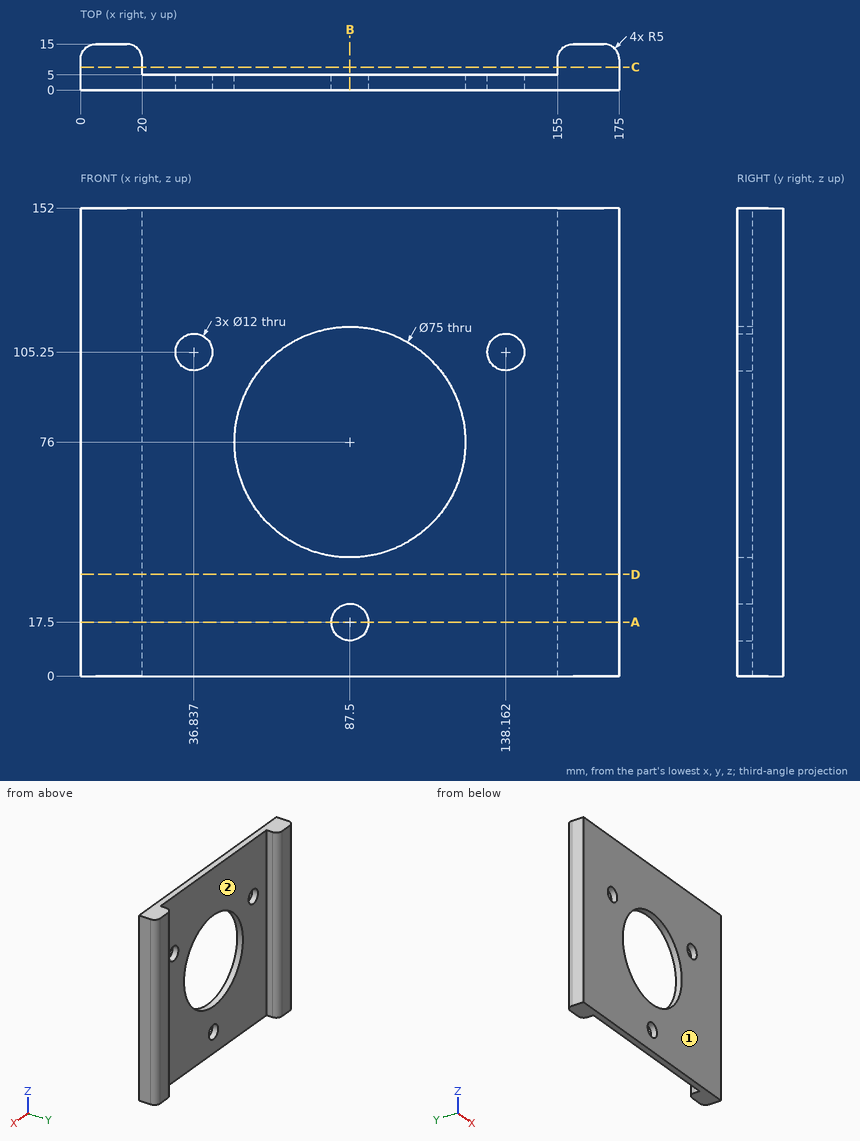
Answer from the drawing. Dimensions are ordinates in mm from the lowest x, y and z of the part. Coordinates: 2 decimals unless noted, no trailing zeros. Write each loop counter-clockwise with the first axis right and the second up, starting at its lowest first coordinate (ties: lowest second). Pieces come first, ordered by that corner, then holes. Notation, with made-up numbers: (15, 21) - (42, 21) arc R9 cw to (42, 31) - close; hole circle Ø8 at (-12.75, -28.5). An arc over 180 degrees is marked (long way). Return JSON: item names as keys, results as strings. Group by question number.
Q1. The part is cut by section D-D on z = 33. Write down the section's boundary in (x, y), and give its area (3 significant figures).
Q2. Find the intervals of material crossed by line 1 along Z through (x, y) = (87.5, 2.9); line 2 along X through (y, z) = (2.85, 105.25) (1 decimal); line 3 along X through (y, z) = (3.3, 17.5), in increasing order. Write a range as [from, to].
Q3. The part is cut by section B-B on x = 87.5. Write down the section's boundary in (y, z).
Q4. For a pull along X with two mould halves and no side action, classify the marked faces 1 and 2 as +X half, -X half, draft (parallel to the pull), parting line (faces both ways), or undercut.
Q5. The part is cut by section C-C on y = 7.5. Write down the section's boundary in (x, z).
Q6. The part is cut by section A-A on z = 17.5. Write down the section's boundary in (x, y), and give its area (3 significant figures).
Q7. Flat-ended cylindrical pins translate along their axes: pin 1 Ø15.5 at (x, z) = (138.16, 105.25) entering from +Y; pin 2 Ø9.5 at (x, z) = (36.84, 105.25) entering from -Y. Find the tip coordinate at first contact, or state that the pin passes through.
Evaluation:
{
 "1": {"outline": "(0, 0) - (175, 0) - (175, 10) arc R5 ccw to (170, 15) - (160, 15) arc R5 ccw to (155, 10) - (155, 5) - (20, 5) - (20, 10) arc R5 ccw to (15, 15) - (5, 15) arc R5 ccw to (0, 10) - close", "area": "1,250 mm2"},
 "2": {"line 1": "z = [0, 11.5], [23.5, 38.5], [113.5, 152]", "line 2": "x = [0, 30.8], [42.8, 64], [111, 132.2], [144.2, 175]", "line 3": "x = [0, 81.5], [93.5, 175]"},
 "3": {"outline": "(0, 0) - (5, 0) - (5, 11.5) - (0, 11.5) - close; (0, 23.5) - (5, 23.5) - (5, 38.5) - (0, 38.5) - close; (0, 113.5) - (5, 113.5) - (5, 152) - (0, 152) - close"},
 "4": {"face 1": "draft", "face 2": "undercut"},
 "5": {"outline": "(0, 0) - (20, 0) - (20, 152) - (0, 152) - close; (155, 0) - (175, 0) - (175, 152) - (155, 152) - close"},
 "6": {"outline": "(0, 0) - (81.5, 0) - (81.5, 5) - (20, 5) - (20, 10) arc R5 ccw to (15, 15) - (5, 15) arc R5 ccw to (0, 10) - close; (93.5, 0) - (175, 0) - (175, 10) arc R5 ccw to (170, 15) - (160, 15) arc R5 ccw to (155, 10) - (155, 5) - (93.5, 5) - close", "area": "1,190 mm2"},
 "7": {"pin 1": "stops at y = 5", "pin 2": "passes through"}
}
